```python
from build123d import *

# Parameters (mm, degrees)
BOSS_EXTRUDE1_DEPTH = 354.999989271
SKETCH2_R           = 4
BOSS_EXTRUDE2_DEPTH = 22
SKETCH3_R           = 4
BOSS_EXTRUDE3_DEPTH = 22
SKETCH4_R           = 4
BOSS_EXTRUDE4_DEPTH = 22
SKETCH5_R           = 4
BOSS_EXTRUDE5_DEPTH = 22
SKETCH6_R           = 55
BOSS_EXTRUDE6_DEPTH = 382
SKETCH8_W           = 20
SKETCH8_H           = 50
CUT_EXTRUDE1_DEPTH  = 10
MOVE_FACE1_BY       = 15
MOVE_FACE1_2_BY     = 15


with BuildPart() as part:
    # Sketch1 → Boss-Extrude1 (new body)
    with BuildSketch(Plane(origin=(354.999989271, 0, 0), x_dir=(0, 0, -1), z_dir=(1, 0, 0))):
        Polygon((-32.00000152, 460.000008345), (-86.999997497, 460.000008345), (-86.999997497, 194.999992847), (-105.999998748, 194.999992847), (-105.999998748, 94.999998808), (-86.999997497, 94.999998808), (-86.999997497, 0), (-32.00000152, 0), align=None)
    extrude(amount=-BOSS_EXTRUDE1_DEPTH)

    # Sketch2 → Boss-Extrude2 (add)
    with BuildSketch(Plane(origin=(354.999989271, 0, 0), x_dir=(0, 0, -1), z_dir=(1, 0, 0))):
        with Locations((-50.00000152, 345.000008345)):
            Circle(SKETCH2_R)
    extrude(amount=BOSS_EXTRUDE2_DEPTH)

    # Sketch3 → Boss-Extrude3 (add)
    with BuildSketch(Plane(origin=(354.999989271, 0, 0), x_dir=(0, 0, -1), z_dir=(1, 0, 0))):
        with Locations((-50.00000152, 115)):
            Circle(SKETCH3_R)
    extrude(amount=BOSS_EXTRUDE3_DEPTH)

    # Sketch4 → Boss-Extrude4 (add)
    with BuildSketch(Plane.ZY):
        with Locations(Location((50.00000152, 115, 0), (0, 0, 180))):
            Circle(SKETCH4_R)
    extrude(amount=BOSS_EXTRUDE4_DEPTH)

    # Sketch5 → Boss-Extrude5 (add)
    with BuildSketch(Plane.ZY):
        with Locations(Location((50.00000152, 345.000008345, 0), (0, 0, 180))):
            Circle(SKETCH5_R)
    extrude(amount=BOSS_EXTRUDE5_DEPTH)

    # Sketch6 → Boss-Extrude6 (add)
    with BuildSketch(Plane.XY.offset(105.999998748)):
        with Locations(Location((177.5, 144.999998808, 0), (0, 0, 114.619992233))):
            Circle(SKETCH6_R)
    extrude(amount=BOSS_EXTRUDE6_DEPTH)

    # Sketch8 → Cut-Extrude1 (cut)
    with BuildSketch(Plane.XY.offset(487.999998748)):
        with Locations((177.5, 144.999998808)):
            Rectangle(SKETCH8_W, SKETCH8_H)
    extrude(amount=-CUT_EXTRUDE1_DEPTH, mode=Mode.SUBTRACT)

    # Move Face1: a face moved outward by 15.0
    extrude(part.faces().sort_by_distance((177.5, 169.999998808, 482.999998748))[0], amount=MOVE_FACE1_BY, dir=(0, -1, 0))

    # Move Face1 2: a face moved outward by 15.0
    extrude(part.faces().sort_by_distance((177.5, 119.999998808, 482.999998748))[0], amount=MOVE_FACE1_2_BY, dir=(0, 1, 0))


solid = part.part
```
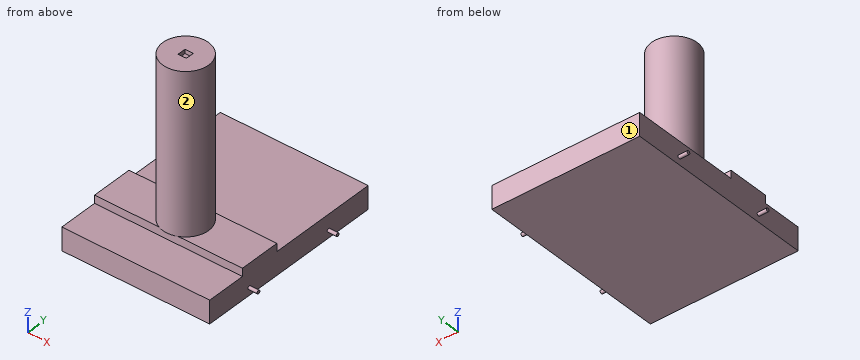
The model under review builds one solid part; all positions refer to its coordinate system, in mm. Face numbers are marked on the shaded views. A direction names the side the tool comes from. Round coordinates to 2 decimals unless told otherwise and drop trailing zeros. Loops run counter-clockwise (first coordinate to the right, second up) from the corner with the lowest first, then second, coordinate; pieces in that order, holes last.
Item 1: Take a section at B-B (z = 162). Write out the cut boundary in (x, y), then the cut area to 3 significant figures.
Determined:
outline: circle Ø110 at (177.5, 145)
area: 9,500 mm2
Item 2: Take a section at C-C (x = 58.5). Write out the cut boundary in (y, z), then the cut area to 3 significant figures.
Determined:
outline: (0, 32) - (460, 32) - (460, 87) - (195, 87) - (195, 106) - (95, 106) - (95, 87) - (0, 87) - close
area: 27,200 mm2
Item 3: Take a section at A-A (x = 177.5). Write out the cut boundary in (y, z), then the cut area to 3 significant figures.
Determined:
outline: (0, 32) - (460, 32) - (460, 87) - (195, 87) - (195, 106) - (200, 106) - (200, 488) - (155, 488) - (155, 478) - (135, 478) - (135, 488) - (90, 488) - (90, 106) - (95, 106) - (95, 87) - (0, 87) - close
area: 69,000 mm2
Item 4: Clearance check with flat-ended pins moving along their axes: pin 1 Ø10 at (x, y) = (257, 146) entering from +Z; pin 2 Ø15 at (x, z) = (214.5, 96.5) entering from -Y; pin 3 Ø5 at (x, z) = (179, 482) entering from +Y. State where each tip first meets the part, or that it passes through.
Determined:
pin 1: stops at z = 106
pin 2: stops at y = 95
pin 3: stops at y = 200
Item 5: For line 1 (Z direction, x = 169, y = 34); line 2 (Z direction, x = 47, y = 191.5); line 3 (Y direction, x = 295, z = 93.5), list the stretches that pass through material, from the lowest coordinate up.
Determined:
line 1: z = 32 to 87
line 2: z = 32 to 106
line 3: y = 95 to 195
Item 6: Take a section at D-D (y = 371). Write out the cut boundary in (x, z), then the cut area to 3 significant figures.
Determined:
outline: (0, 32) - (355, 32) - (355, 87) - (0, 87) - close
area: 19,500 mm2
Item 7: For the marked faces 1 and 2, list the 3-axis set-ups (+Z, -Z, +X, -X, +Y, -Y) from which the entire face can be reached by the end or side of a thin tool; tool diameter is ignored.
Determined:
face 1: +Z, -Z, +X, -X, +Y
face 2: +Z
